from build123d import *

# Parameters (mm, degrees)
F0_R     = 25
F1_DEPTH = 1
F5_R     = 25
F5_R_2   = 23.25
F6_DEPTH = 3.2
F7_R     = 0.9


with BuildPart() as f1:
    # F0 (on Top) → F1 (new body)
    with BuildSketch(Plane.XY):
        Circle(F0_R)
    extrude(amount=F1_DEPTH)

    # F3 (on Front) → F4 (revolve)
    with BuildSketch(Plane.XZ):
        Polygon((21, 1), (23.25, 1), (23.25, 5.6), (21.8255799264, 5.6), align=None)
    revolve(axis=Axis((0, 0, 1), (0, 0, 1)))

    # F5 (on face) → F6 (join)
    with BuildSketch(Plane.XY.offset(1)):
        Circle(F5_R)
        Circle(F5_R_2, mode=Mode.SUBTRACT)
    extrude(amount=F6_DEPTH)

    # F7
    f7_edges = [f1.edges().sort_by_distance(p)[0] for p in [
        (-21.82558, 0, 5.6),
    ]]
    fillet(f7_edges, radius=F7_R)


solid = f1.part
Source: CAD feature listing. Evaluate the final solid. Frame: model axes, mm. A direction names the side the tool comes from. Give positions to 0.01 mm unless a question says otherwise; leave off trailing zeros. Write each loop counter-clockwise with the first axis right and the second up, starting at its lowest first coordinate (ties: lowest second). Pieces come first, ordered by that corner, then holes. Notation, with made-up numbers: M -18.75,-7 L -12.75,-7 A21 cw -12.75,19 Z; hole C 67,56.5 d1. An arc over 180 degrees is marked long. Answer as a JSON object with one key per item and string values.
Q1. Ray query, line 1 along Z through (x, y) = (17.5, 7); line 2 along Y through (x, z) = (5.5, 1.4); line 3 along X through (y, z) = (9.5, 1.5). Return the intervals inside material, ascending.
Geometry check:
{"line 1": "z = 0 to 1", "line 2": "y = -24.39 to -20.34, 20.34 to 24.39", "line 3": "x = -23.12 to -18.83, 18.83 to 23.12"}
Q2. Cut plane A-A, the plane y = 0. Return the cut outline in (x, z).
Geometry check:
{"outline": "M -25,0 L 25,0 L 25,4.2 L 23.25,4.2 L 23.25,5.6 L 22.58,5.6 A0.9 ccw 21.69,4.86 L 21,1 L -21,1 L -21.69,4.86 A0.9 ccw -22.58,5.6 L -23.25,5.6 L -23.25,4.2 L -25,4.2 Z"}
Q3. Mould query, pull axis Y, two halves, no side actions, for faces 1 (the face through (-2.738, 20.855, 1.187)), 2 (the face through (22.176, 6.984, 4.91)), 3 (the face through (17, -17, 4.2)). Classes: +Y half, -Y half, draft (parallel to the pull), parting line (faces both ways), or undercut.
Geometry check:
{"face 1": "undercut", "face 2": "parting line", "face 3": "draft"}
Q4. Cut plane C-C, the plane z = 1.7. Return the cut outline in (x, y), then the cut area to 3 significant figures.
Geometry check:
{"outline": "C 0,0 d50; hole C 0,0 d42.25", "area": "561 mm^2"}
Q5. Access query for faces 4 (the face through (0, 0, 1)), 5 (the face through (23.846, 7.509, 2.071)). Directions: +Z, -Z, +X, -X, +Y, -Y. A direction counts if a zero-diameter tool reaches every point of the face in a straight line with its end or side. Return the directions, or none.
Geometry check:
{"face 4": "+Z", "face 5": "+Z, -Z"}
Q6. Contact query for flat-ended pins moving along their axis: P1, Ø2, axis at y = 4.5, z = 4, coming from the +X side; P2, Ø1, axis at y = 11.5, z = 4, coming from the -X side; P3, Ø3, axis at x = 0.5, z = 3.5, coming from the +Y side. Output: stop coordinate, or through.
Geometry check:
{"P1": "stops at x = 24.75", "P2": "stops at x = -22.45", "P3": "stops at y = 25"}
